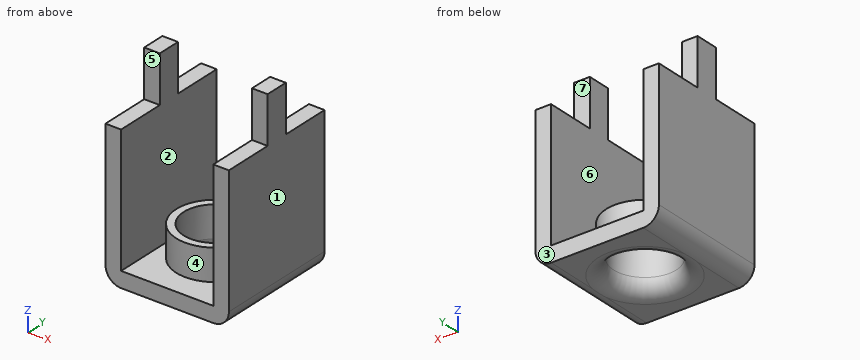
```python
from build123d import *

# Parameters (mm, degrees)
SKETCH_1_W      = 7.9
SKETCH_1_H      = 7.9
SKETCH_1_R      = 2
EXTRUDE_1_DEPTH = 1
SKETCH_2_W      = 1
SKETCH_2_H      = 7.9
EXTRUDE_2_DEPTH = 9.2
SKETCH_3_W      = 1
SKETCH_3_H      = 1.5
EXTRUDE_3_DEPTH = 3
SKETCH_4_R      = 2.480212027
SKETCH_4_R_2    = 2
EXTRUDE_4_DEPTH = 2
FILLET_2_R      = 1


with BuildPart() as part:
    # 草图1 → 凸台-拉伸1 (new body)
    with BuildSketch(Plane.XY):
        Rectangle(SKETCH_1_W, SKETCH_1_H)
        Circle(SKETCH_1_R, mode=Mode.SUBTRACT)
    extrude(amount=EXTRUDE_1_DEPTH)

    # 草图2 → 凸台-拉伸2 (add)
    with BuildSketch(Plane.XY):
        with Locations((-3.45, 0)):
            Rectangle(SKETCH_2_W, SKETCH_2_H)
        with Locations((3.45, 0)):
            Rectangle(SKETCH_2_W, SKETCH_2_H)
    extrude(amount=EXTRUDE_2_DEPTH)

    # 草图3 → 凸台-拉伸3 (add)
    with BuildSketch(Plane.XY.offset(9.2)):
        with Locations((-3.45, 0)):
            Rectangle(SKETCH_3_W, SKETCH_3_H)
        with Locations((3.45, 0)):
            Rectangle(SKETCH_3_W, SKETCH_3_H)
    extrude(amount=EXTRUDE_3_DEPTH)

    # 草图4 → 凸台-拉伸4 (add)
    with BuildSketch(Plane.XY.offset(1)):
        with Locations(Location((0, 0, 0), (0, 0, 180))):
            Circle(SKETCH_4_R)
        Circle(SKETCH_4_R_2, mode=Mode.SUBTRACT)
    extrude(amount=EXTRUDE_4_DEPTH)

    # 圆角2
    # the kernel refuses this fillet: 1 mm, written as the material it takes off along each edge
    with BuildSketch(Plane(origin=(0, 0, 0), x_dir=(1, 0, 0), z_dir=(0, -1, 0))) as fillet_2_piece_1:
        with BuildLine():
            CenterArc((2 + FILLET_2_R, FILLET_2_R), FILLET_2_R, 180, 90)
            Line((2 + FILLET_2_R, 0), (2, 0))
            Line((2, 0), (2, FILLET_2_R))
        make_face()
    revolve(axis=Axis((0, 0, 0), (0, 0, 1)), mode=Mode.SUBTRACT)
    with BuildSketch(Plane(origin=(-3.95, 6.45, 0), x_dir=(0, 0, 1), z_dir=(0, -1, 0)), Plane(origin=(3.95, -6.45, 0), x_dir=(0, 0, 1), z_dir=(0, 1, 0))) as fillet_2_piece_2:
        with BuildLine():
            CenterArc((FILLET_2_R, -FILLET_2_R), FILLET_2_R, 90, 90)
            Line((0, -FILLET_2_R), (0, 0))
            Line((0, 0), (FILLET_2_R, 0))
        make_face()
    extrude(amount=12.9, mode=Mode.SUBTRACT)


solid = part.part
```
Verification items for the finished model (mm, model axes). Face numbers are marked on the shaded views. A direction names the side the tool comes from. Round coordinates to 2 decimals unless told otherwise and drop trailing zeros. Loops run counter-clockwise (first coordinate to the right, second up) from the corner with the lowest first, then second, coordinate; pieces in that order, holes last. Notation, with made-up numbers: (-37.5, 70) -> (-7.5, 70) arc R22 ccw to (-7.5, 107) -> close; hole circle Ø2 at (-9, 25.5). An arc over 180 degrees is marked (long way). Answer as a JSON object with one key per item and string values.
Q1. Section check C-C (z = 11). Record the boundary of the cut face in (x, y).
Data:
{"outline": "(-3.95, -0.75) -> (-2.95, -0.75) -> (-2.95, 0.75) -> (-3.95, 0.75) -> close; (2.95, -0.75) -> (3.95, -0.75) -> (3.95, 0.75) -> (2.95, 0.75) -> close"}
Q2. Section check B-B (x = 0). Record the boundary of the cut face in (y, z).
Data:
{"outline": "(-3.95, 0) -> (-3, 0) arc R1 ccw to (-2, 1) -> (-2, 3) -> (-2.48, 3) -> (-2.48, 1) -> (-3.95, 1) -> close; (2, 1) arc R1 ccw to (3, 0) -> (3.95, 0) -> (3.95, 1) -> (2.48, 1) -> (2.48, 3) -> (2, 3) -> close"}
Q3. Access from +Z, -Z, +X, -X, +Y, -Y to the whole of each face (thin tool, end or side, straight path). Record for the marked faces 4, 5, 6 and 7.
Data:
{"face 4": "+Z", "face 5": "+Z, +X, -X, -Y", "face 6": "+Z, +Y, -Y", "face 7": "+Z, +X, -X, +Y"}
Q4. Section check A-A (z = 2.75). Record the boundary of the cut face in (x, y), then the cut area to 3 significant figures.
Data:
{"outline": "(-3.95, -3.95) -> (-2.95, -3.95) -> (-2.95, 3.95) -> (-3.95, 3.95) -> close; circle Ø4.96 at (0, 0); (2.95, -3.95) -> (3.95, -3.95) -> (3.95, 3.95) -> (2.95, 3.95) -> close; hole circle Ø4 at (0, 0)", "area": "22.6 mm2"}
Q5. Go/stop test with flat-tipped pins: P1, Ø0.5, axis at x = 3.5, z = 11.5, coming from the +Y side; P2, Ø0.8, axis at x = -3.5, y = 3, coming from the +Z side; P3, Ø1, axis at x = 1, y = -1, coming from the +Z side; P4, Ø0.5, axis at x = -3.5, z = 10, coming from the -Y side. Record where each tip stops, or that it passes through.
Data:
{"P1": "stops at y = 0.75", "P2": "stops at z = 9.2", "P3": "passes through", "P4": "stops at y = -0.75"}
Q6. Section check D-D (y = 0). Record the boundary of the cut face in (x, z) (3 decimals), then the cut area to 3 significant figures.
Data:
{"outline": "(-3.95, 1) arc R1 ccw to (-2.975, 0) arc R1 ccw to (-2, 1) -> (-2, 3) -> (-2.48, 3) -> (-2.48, 1) -> (-2.95, 1) -> (-2.95, 12.2) -> (-3.95, 12.2) -> close; (2, 1) arc R1 ccw to (2.975, 0) arc R1 ccw to (3.95, 1) -> (3.95, 12.2) -> (2.95, 12.2) -> (2.95, 1) -> (2.48, 1) -> (2.48, 3) -> (2, 3) -> close", "area": "27.4 mm2"}
Q7. Draft check along X on the marked faces 1, 2 and 3. Enter one of: pulls with the +X half, pulls with the -X half, needs draft (parallel to the pull), parting line crosses it, or undercut.
Data:
{"face 1": "pulls with the +X half", "face 2": "undercut", "face 3": "needs draft"}
Q8. Scan lines: line 1 (Y direction, x = 0, z = 2.3); line 2 (X direction, y = 0.75, z = 4); line 3 (Y direction, x = -3, z = 10.75). Record each from-to range of solid material in increasing order. Write a range as from..to.
Data:
{"line 1": "y = -2.48..-2, 2..2.48", "line 2": "x = -3.95..-2.95, 2.95..3.95", "line 3": "y = -0.75..0.75"}
